Geometry check sheet. Reference: the model listing, model coordinates, mm. A direction names the side the tool comes from. Give positions to 0.01 mm unless a question says otherwise; leave off trailing zeros. Write each loop counter-clockwise with the first axis right and the second up, starting at its lowest first coordinate (ties: lowest second). Pieces come first, ordered by that corner, then holes. Notation, with made-up numbers: (86.5, 30.25) -> (144.5, 30.25) arc R11 ccw to (144.5, 40.25) -> close; hole circle Ø4 at (22, 38). An arc over 180 degrees is marked (long way). Write item = value, one per line. Start each with the question number.
1. Set-up check for faces 4 (the flat face through (-24, 2.5, 0)), 5 (the cylindrical face through (-28.5, 0, -8)), 6 (the flat face through (22, 0, 6)): record each of +Z, -Z, +X, -X, +Y, -Y from which the full face is reachable in a straight line by a thin tool's end or side.
2. Cross-section at A-A, the plane y = 3.5. Record the cut outline in (x, z).
3. Cross-section at C-C, the plane x = 25.5. Record the cut outline in (y, z).
4. Mould release check, pull along X, two halves, no side actions. Record for faces 1 (the flat face through (24.127, 0, -1)), 2 (the flat face through (-6.5, 4, 3)), 3 (the flat face through (-20, 0, 4.824)): pulls with the +X half, pulls with the -X half, needs draft (parallel to the pull), parting line crosses it, or undercut.
5. Cross-section at B-B, the plane y = 0.5. Record the cut outline in (x, z).
6. Depth check by flat-ended pin: P1, Ø2.5, axis at x = -24.5, y = 0, coming from the +Z side; P2, Ø7.5, axis at x = -28.37, z = -2, coming from the -Y side; P3, Ø2.5, axis at x = 16, y = 0, coming from the +Z side; P4, Ø6, axis at x = 30.13, z = -2, coming from the -Y side. Enter the tip coordinate at first touch or a pass-through.
7. Thickness scan on line 1 along X through (y, z) = (3.75, 22); line 2 along Z through (x, y) = (-20.5, -1.75); line 3 along Y through (x, z) = (26, -4.5). Record the ranges inside material, lowest first.
```python
from build123d import *

# Parameters (mm, degrees)
F0_W     = 10
F0_H     = 15
F1_DEPTH = 25.2
F4_R     = 4.25
F5_DEPTH = 25
F6_R     = 3.2
F7_DEPTH = 2.5
F8_SIZE  = 3


with BuildPart() as f1:
    # F0 (on Top) → F1 (new body)
    with BuildSketch(Plane.XY):
        Rectangle(F0_W, F0_H)
    extrude(amount=F1_DEPTH)

    # F4 (on line) → F5 (cut)
    with BuildSketch(Plane(origin=(10.0907595655, 0, 2.2370675377), x_dir=(0, 1, 0), z_dir=(0.9762960071, 0, 0.2164396139))):
        with Locations((0, 16.9178019303)):
            Circle(F4_R)
    extrude(amount=-F5_DEPTH, mode=Mode.SUBTRACT)

    # F6 (on Front) → F7 (join, symmetric)
    with BuildSketch(Plane.XZ):
        with BuildLine():
            ThreePointArc((-34.3731079698, -2), (-28.3731079698, -8), (-22.3731079698, -2))
            ThreePointArc((-22.3731079698, -2), (-28.3731079698, 4), (-34.3731079698, -2))
        make_face()
        with Locations((-28.3731079698, -2)):
            Circle(F6_R, mode=Mode.SUBTRACT)
        with BuildLine():
            ThreePointArc((-34.3731079698, -2), (-28.3731079698, 4), (-22.3731079698, -2))
            Line((-22.3731079698, -2), (-22.3731079698, 0))
            Line((-22.3731079698, 0), (24.1268920302, 0))
            Line((24.1268920302, 0), (24.1268920302, -2))
            ThreePointArc((24.1268920302, -2), (30.1268920302, 4), (36.1268920302, -2))
            Line((36.1268920302, -2), (36.1268920302, 3.4847958965))
            Line((36.1268920302, 3.4847958965), (36.1268920302, 6))
            Line((36.1268920302, 6), (4.5456811786, 6))
            Line((4.5456811786, 6), (4.3161994133, 4.8236340731))
            Line((4.3161994133, 4.8236340731), (-34.3731079698, 4.8236340731))
            Line((-34.3731079698, 4.8236340731), (-34.3731079698, 3.4847958965))
            Line((-34.3731079698, 3.4847958965), (-34.3731079698, -2))
        make_face()
        with BuildLine():
            ThreePointArc((36.1268920302, -2), (30.1268920302, 4), (24.1268920302, -2))
            ThreePointArc((24.1268920302, -2), (30.1268920302, -8), (36.1268920302, -2))
        make_face()
        with Locations((30.1268920302, -2)):
            Circle(F6_R, mode=Mode.SUBTRACT)
    extrude(amount=F7_DEPTH, both=True)

    # F8
    f8_edges = [f1.edges().sort_by_distance(p)[0] for p in [
        (-5, 0, 4.823634),
        (5, 0, 6),
        (0, -7.5, 25.2),
        (0, 7.5, 25.2),
        (5, -2.5, 3),
        (5, 2.5, 3),
        (-5, 2.5, 2.411817),
        (-5, -2.5, 2.411817),
        (-34.373108, 0, 4.823634),
    ]]
    chamfer(f8_edges, length=F8_SIZE)


solid = f1.part
```
Answers:
q1.face_4 = +Z, -Z, -X, +Y
q1.face_5 = -Z, +Y, -Y
q1.face_6 = +Z, +X, +Y, -Y
q2.outline = (-7, 0) -> (7, 0) -> (7, 7) -> (5, 9) -> (5, 15.97) -> (-5, 13.75) -> (-5, 7.82) -> (-7, 5.82) -> close; (-5, 18.69) -> (5, 20.91) -> (5, 25.2) -> (-5, 25.2) -> close
q3.outline = (-2.5, -5.82) -> (2.5, -5.82) -> (2.5, 6) -> (-2.5, 6) -> close
q4.face_1 = undercut
q4.face_2 = pulls with the -X half
q4.face_3 = needs draft
q5.outline = (-34.37, -2) arc R6 ccw to (-22.37, -2) -> (-22.37, 0) -> (24.13, 0) -> (24.13, -2) arc R6 ccw to (36.13, -2) -> (36.13, 6) -> (8, 6) -> (5, 9) -> (5, 14.11) -> (-5, 11.9) -> (-5, 7.82) -> (-8, 4.82) -> (-31.37, 4.82) -> (-34.37, 1.82) -> close; (-5, 20.54) -> (5, 22.76) -> (5, 25.2) -> (-5, 25.2) -> close; hole circle Ø6.4 at (-28.37, -2); hole circle Ø6.4 at (30.13, -2)
q6.P1 = 4.82
q6.P2 = -2.5
q6.P3 = 6
q6.P4 = through
q7.line_1 = -5 to 5
q7.line_2 = 0 to 4.82
q7.line_3 = -2.5 to 2.5
